```python
from build123d import *

# Parameters (mm, degrees)
SKETCH2_R           = 20
BOSS_EXTRUDE1_DEPTH = 20
BOSS_EXTRUDE2_DEPTH = 25
CUT_EXTRUDE1_DEPTH  = 172.537167984
RIB1_REACH          = 173.537
SKETCH5_WALL_W      = 396.064531104
SKETCH5_WALL_H      = 10
HOLE1_D             = 20
HOLE1_DEPTH         = 25
HOLE1_CBORE_D       = 40
HOLE1_CBORE_DEPTH   = 10


with BuildPart() as part:
    # Sketch1 → Revolve1 (revolve)
    with BuildSketch(Plane(origin=(0, 0, 0), x_dir=(0, 0, -1), z_dir=(1, 0, 0)), mode=Mode.PRIVATE) as revolve1_sk:
        Polygon((0, 30), (0, 40), (70, 58.75644347), (70, 48.75644347), align=None)
    revolve(revolve1_sk.sketch.rotate(Axis((0, 0, 0), (0, 0, -1)), 90), axis=Axis((0, 0, 0), (0, 0, -1)))

    # Sketch2 → Boss-Extrude1 (add)
    with BuildSketch(Plane(origin=(0, 0, -70), x_dir=(-1, 0, 0), z_dir=(0, 0, -1))):
        with BuildLine():
            Line((90, -90), (-90, -90))
            Line((-90, -90), (-56.03473707, 17.675629856))
            ThreePointArc((-56.03473707, 17.675629856), (0, 58.75644347), (56.03473707, 17.675629856))
            Line((56.03473707, 17.675629856), (90, -90))
        make_face()
        Circle(SKETCH2_R, mode=Mode.SUBTRACT)
    extrude(amount=BOSS_EXTRUDE1_DEPTH)

    # Sketch3 → Boss-Extrude2 (add)
    with BuildSketch(Plane.XZ.offset(90)):
        with BuildLine():
            Line((-90, -90), (90, -90))
            Line((90, -90), (90, -10))
            ThreePointArc((90, -10), (84.142135624, 4.142135624), (70, 10))
            Line((70, 10), (-70, 10))
            ThreePointArc((-70, 10), (-84.142135624, 4.142135624), (-90, -10))
            Line((-90, -10), (-90, -90))
        make_face()
    extrude(amount=BOSS_EXTRUDE2_DEPTH)

    # Sketch4 → Cut-Extrude1 (cut, through all)
    with BuildSketch(Plane(origin=(0, 0, 0), x_dir=(1, 0, 0), z_dir=(0, 1, 0))):
        with BuildLine():
            Line((-10, -30), (-10, 30))
            ThreePointArc((-10, 30), (0, 40), (10, 30))
            Line((10, 30), (10, -30))
            ThreePointArc((10, -30), (0, -40), (-10, -30))
        make_face()
    extrude(amount=CUT_EXTRUDE1_DEPTH, mode=Mode.SUBTRACT)

    # Sketch5 wall → Rib1 (add, up to next)
    with BuildSketch(Plane(origin=(0, -65, 5), x_dir=(0, 0.980580675691, -0.196116135138), z_dir=(0, 0.196116135138, 0.980580675691)), mode=Mode.PRIVATE) as rib1_sk1:
        Rectangle(SKETCH5_WALL_W, SKETCH5_WALL_H)
    rib1_tool1 = extrude(rib1_sk1.sketch, amount=-RIB1_REACH, mode=Mode.PRIVATE) - part.part
    add(rib1_tool1.solids().sort_by_distance((0, -65, 5))[0])

    # Hole1
    with Locations(Plane(origin=(0, -90, 0), x_dir=(1, 0, 0), z_dir=(0, 1, 0))):
        with Locations((50, 30)):
            hole1 = CounterBoreHole(HOLE1_D / 2, HOLE1_CBORE_D / 2, HOLE1_CBORE_DEPTH, depth=HOLE1_DEPTH)

    # Mirror1: Hole1 across plane
    add(hole1.mirror(Plane(origin=(0, 0, 0), x_dir=(0, 0, 1), z_dir=(1, 0, 0))), mode=Mode.SUBTRACT)


solid = part.part
```
Could you check a few things on this model? Use its own coordinates, in mm. A direction names the side the tool comes from. Round coordinates to 2 decimals unless told otherwise and drop trailing zeros. Loops run counter-clockwise (first coordinate to the right, second up) from the corner with the lowest first, then second, coordinate; pieces in that order, holes last. Notation, with made-up numbers: M 76.5,46 L 114.5,46 A21 cw 114.5,61 Z; hole C -16,29.5 d5. An arc over 180 degrees is marked long. Put each result on its own line as item: value.
Q1. Imagine slicing it at B-B (y = -77). Write out the boundary of the cut face in (x, z).
Check result:
outline: M -85.9,-90 L 85.9,-90 L 85.9,-70 L 5,-70 L 5,7.4 L -5,7.4 L -5,-70 L -85.9,-70 Z
Q2. For pin 1 (18 mm diameter, centred on x = -50, z = -30, fed in from -Y); pin 2 (5 mm diameter, centred on y = -11, z = -74.5, fed in from +X); pin 3 (16 mm diameter, centred on x = 50, z = -30, fed in from -Y), each with a flat end and sliding along its axis, tell me the tip position at first contact or that it passes through.
Check result:
pin 1: y = -25.74
pin 2: x = 65.87
pin 3: y = -23.98
Q3. I need wall thicknesses on probe 1 along Y at (x, z) = (-12.5, -34.5); probe 2 along Y at (x, z) = (-31, -53); probe 3 along Z at (x, y) = (50, -97). Which ranges of each line are inside material? Lowest first, please.
Check result:
probe 1: -115 to -90, -47.63 to -37.2, 37.2 to 47.63
probe 2: -115 to -90, -44.46 to -31.51, 31.51 to 44.46
probe 3: -90 to -50, -10 to 10
Q4. Imagine slicing it at A-A (z = -80.5). Write out the boundary of the cut face in (x, y), then the cut area to 3 significant figures.
Check result:
outline: M -90,-115 L 90,-115 L 90,-90 L 56.03,17.68 A58.76 ccw -56.03,17.68 L -90,-90 Z; hole C 0,0 d40
area: 22,300 mm2
Q5. Imagine slicing it at D-D (z = -43). Write out the boundary of the cut face in (x, y).
Check result:
outline: M -90,-115 L 90,-115 L 90,-90 L 65.2,-90 L 65.2,-100 L 34.8,-100 L 34.8,-90 L 5,-90 L 5,-51.28 A51.52 ccw long -5,-51.28 L -5,-90 L -34.8,-90 L -34.8,-100 L -65.2,-100 L -65.2,-90 L -90,-90 Z; hole C 0,0 d83.04
Q6. On a 3-axis mill with a long thin cutter (end or side, diameter ignored), from which of +Z, -Z, +X, -X, +Y, -Y can I reach the whole of each face in a straight line? I mean faces 1 (the face through (-41, -100, -35)), 2 (the face through (-58, -108, -24)), 3 (the face through (0, 44, -40)), 4 (the face through (5, -73, -33)). Say none if no direction works.
Check result:
face 1: none
face 2: -Y
face 3: +Z, +Y
face 4: +Z, +X
Q7. Imagine slicing it at C-C (x = 73). Write out the boundary of the cut face in (y, z), then the cut area to 3 significant figures.
Check result:
outline: M -115,-90 L -36.11,-90 L -36.11,-70 L -90,-70 L -90,9.77 L -115,9.77 Z
area: 3,570 mm2
Q8. Thinking about a two-plate mould opening in Z: for faces 5 (the face through (-1, -46, -90)), 6 (the face through (21, 1, -70)), 7 (the face through (10, 38, -15)), 8 (the face through (6, -30, 0)), which applies, released by +Z, released by -Z, zero draft, split by the parting line, or undercut?
Check result:
face 5: released by -Z
face 6: undercut
face 7: zero draft
face 8: released by +Z
